Check sheet for the modelled part. Datum: model origin and axes. Units: mm. A direction names the side the tool comes from. Round coordinates to 2 decimals unless told otherwise and drop trailing zeros. Loops run counter-clockwise (first coordinate to the right, second up) from the corner with the lowest first, then second, coordinate; pieces in that order, holes last. Notation, with made-up numbers: M 2.5,-39.75 L 55.5,-39.75 A14 cw 55.5,-17.75 Z; hole C 62,22 d1. An arc over 180 degrees is marked long. One line per question, with ' | ' between items. Start each with the question number.
(1) Go/stop test with flat-tipped pins: P1, Ø5.5, axis at y = -8.5, z = 51.5, coming from the -X side; P2, Ø11.5, axis at x = 59, y = -8, coming from the -Z side; P3, Ø11.5, axis at x = 57, y = -18, coming from the +Z side. Record where each tip stops, or that it passes through.
(2) Draft check along X on faces 4 (the face through (12.5, 0, -3.7)), 5 (the face through (-12.653, -13, 49)), 6 (the face through (11.581, -13, 49)), 7 (the face through (54.295, -13, -2)). Enter one of: +X half, -X half, draft (parallel to the pull), parting line (faces both ways), or undercut.
(3) Thickness scan on probe 1 along X at (y, z) = (-23.25, -34); probe 2 along X at (y, z) = (-22, 15) (3 decimals); probe 3 along Z at (x, y) = (25, -15.25). Record the ranges inside material, lowest first. Write a range as [from, to].
(4) Section check A-A (z = 0). Record the boundary of the cut face in (x, y).
(5) Section check D-D (y = -22.5). Record the boundary of the cut face in (x, z), and give its area (3 significant figures).
(6) Tool access check on faces 1 (the face through (-62, -13, -10.086)), 2 (the face through (0, -13, 43.451)), 3 (the face through (2, -13, -52.072)). Record the directions out of +Z, -Z, +X, -X, +Y, -Y that give a thin tool (end or side, any length) a straight path to the whole face; none if there is none.
(7) Section check C-C (z = -36.5). Record the boundary of the cut face in (x, y).
(8) Section check B-B (x = 0). Record the boundary of the cut face in (y, z), and give its area (3 significant figures).
```python
from build123d import *

# Parameters (mm, degrees)
F0_R     = 12.683185
F0_R_2   = 12.629116
F1_DEPTH = 25.4


with BuildPart() as f1:
    # F0 (on Front) → F1 (new body)
    with BuildSketch(Plane.XZ):
        with BuildLine():
            Line((54.29461, -10.215261), (54.29461, 6.396934))
            Line((54.29461, 6.396934), (64.678587, 6.396934))
            ThreePointArc((64.678587, 6.396934), (47.894565, 41.329487), (11.581181, 54.869236))
            Line((11.581181, 54.869236), (11.581181, 43.450589))
            Line((11.581181, 43.450589), (-12.652815, 43.450589))
            Line((-12.652815, 43.450589), (-12.652815, 54.911602))
            ThreePointArc((-12.652815, 54.911602), (-49.127425, 42.752813), (-67.202314, 8.818588))
            Line((-67.202314, 8.818588), (-56.818337, 8.818588))
            Line((-56.818337, 8.818588), (-56.818337, -10.085616))
            Line((-56.818337, -10.085616), (-67.202314, -10.085616))
            ThreePointArc((-67.202314, -10.085616), (-49.926198, -50.996741), (-7.323014, -63.532812))
            Line((-7.323014, -63.532812), (-7.323014, -52.071802))
            Line((-7.323014, -52.071802), (11.581181, -52.071802))
            Line((11.581181, -52.071802), (11.581181, -63.532812))
            ThreePointArc((11.581181, -63.532812), (49.58814, -48.284983), (64.678587, -10.215261))
            Line((64.678587, -10.215261), (54.29461, -10.215261))
        make_face()
        with Locations((-34.668908, -32.428525)):
            Circle(F0_R, mode=Mode.SUBTRACT)
        with Locations((28.988812, -32.428525)):
            Circle(F0_R, mode=Mode.SUBTRACT)
        with Locations((-34.668908, 24.355358)):
            Circle(F0_R, mode=Mode.SUBTRACT)
        Circle(F0_R_2, mode=Mode.SUBTRACT)
        with Locations((28.988812, 24.355358)):
            Circle(F0_R, mode=Mode.SUBTRACT)
    extrude(amount=F1_DEPTH)


solid = f1.part
```
The answers:
1) P1: x = -40.34 | P2: z = -44.2 | P3: z = 37.97
2) face 4: draft | face 5: undercut | face 6: undercut | face 7: +X half
3) probe 1: [-62.5, -47.25], [-22.08, 16.4], [41.57, 59.66] | probe 2: [-66.14, -43.233], [-26.105, 20.425], [37.553, 63.388] | probe 3: [-62.1, -44.47], [-20.39, 12.32], [36.39, 53.46]
4) outline: M -56.82,-25.4 L -12.63,-25.4 L -12.63,0 L -56.82,0 Z; M 12.63,-25.4 L 54.29,-25.4 L 54.29,0 L 12.63,0 Z
5) outline: M -67.2,-10.09 A51.85 ccw -7.32,-63.53 L -7.32,-52.07 L 11.58,-52.07 L 11.58,-63.53 A51.85 ccw 64.68,-10.22 L 54.29,-10.22 L 54.29,6.4 L 64.68,6.4 A51.85 ccw 11.58,54.87 L 11.58,43.45 L -12.65,43.45 L -12.65,54.91 A51.85 ccw -67.2,8.82 L -56.82,8.82 L -56.82,-10.09 Z; hole C -34.67,-32.43 d25.37; hole C -34.67,24.36 d25.37; hole C 0,0 d25.26; hole C 28.99,-32.43 d25.37; hole C 28.99,24.36 d25.37 | area: 9,990 mm²
6) face 1: -X, +Y, -Y | face 2: +Z, +Y, -Y | face 3: -Z, +Y, -Y
7) outline: M -61.26,-25.4 L -46.68,-25.4 L -46.68,0 L -61.26,0 Z; M -22.66,-25.4 L 16.98,-25.4 L 16.98,0 L -22.66,0 Z; M 41,-25.4 L 58.38,-25.4 L 58.38,0 L 41,0 Z
8) outline: M -25.4,-52.07 L 0,-52.07 L 0,-12.63 L -25.4,-12.63 Z; M -25.4,12.63 L 0,12.63 L 0,43.45 L -25.4,43.45 Z | area: 1,780 mm²
